Work out the finished part from the listing and answer in its coordinate system (mm). Face numbers are marked on the shaded views. Give positions to 0.01 mm unless a question says otherwise; leave off trailing zeros. Loops run counter-clockwise (first coordinate to the right, second up) from the corner with the lowest first, then second, coordinate; pieces in that order, holes last. Notation, with made-up numbers: (52, -29) - (93, -29) arc R16 cw to (93, -17) - close; hole circle Ø3 at (41.5, 63.5). An arc over 180 degrees is marked (long way). One line per question, with ' | ' between items.
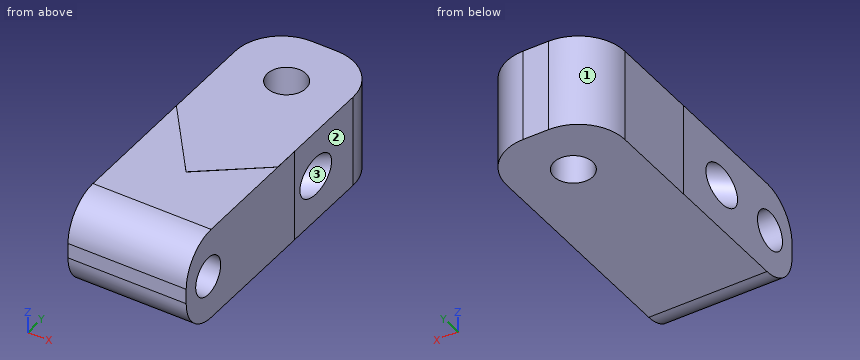
from build123d import *

# Parameters (mm, degrees)
SKETCH5_W           = 60
SKETCH5_H           = 60
SKETCH5_R           = 12.5
BOSS_EXTRUDE3_DEPTH = 25
SKETCH9_R           = 12.5
BOSS_EXTRUDE5_DEPTH = 30
SKETCH10_R          = 12.5
BOSS_EXTRUDE6_DEPTH = 38.21
SKETCH5_2_R         = 12.5
CUT_EXTRUDE2_DEPTH  = 115


with BuildPart() as part:
    # Sketch5 → Boss-Extrude3 (new body, symmetric)
    with BuildSketch(Plane(origin=(0, 0, 0), x_dir=(0, 0, -1), z_dir=(0.789084085, 0.6142852, 0))):
        Rectangle(SKETCH5_W, SKETCH5_H)
        Circle(SKETCH5_R, mode=Mode.SUBTRACT)
    extrude(amount=BOSS_EXTRUDE3_DEPTH, both=True)

    # Sketch9 → Boss-Extrude5 (add, symmetric)
    with BuildSketch(Plane.XY):
        with BuildLine():
            Line((38.155658124, -8.315392543), (38.155658124, 67.179146139))
            ThreePointArc((38.155658124, 67.179146139), (29.368861559, 88.392349575), (8.155658124, 97.179146139))
            Line((8.155658124, 97.179146139), (-8.155658124, 97.179146139))
            ThreePointArc((-8.155658124, 97.179146139), (-29.368861559, 88.392349575), (-38.155658124, 67.179146139))
            Line((-38.155658124, 67.179146139), (-38.155658124, 8.315392543))
            Line((-38.155658124, 8.315392543), (38.155658124, -8.315392543))
        make_face()
        with Locations((0, 59.597275262)):
            Circle(SKETCH9_R, mode=Mode.SUBTRACT)
    extrude(amount=BOSS_EXTRUDE5_DEPTH, both=True)

    # Sketch10 → Boss-Extrude6 (add, symmetric)
    with BuildSketch(Plane(origin=(0, 0, 0), x_dir=(0, 0, -1), z_dir=(1, 0, 0))):
        with BuildLine():
            Line((-4.782552043, -100.050547257), (5, -100.050547257))
            ThreePointArc((5, -100.050547257), (22.67766953, -92.728216787), (30, -75.050547257))
            Line((30, -75.050547257), (30, 8.315392543))
            Line((30, 8.315392543), (-30, 8.315392543))
            Line((-30, 8.315392543), (-29.782467066, -75.115730425))
            ThreePointArc((-29.782467066, -75.115730425), (-22.437160802, -92.751247514), (-4.782552043, -100.050547257))
        make_face()
        with Locations((0.225286959, -78.050547257)):
            Circle(SKETCH10_R, mode=Mode.SUBTRACT)
    extrude(amount=BOSS_EXTRUDE6_DEPTH, both=True)

    # Sketch5_2 → Cut-Extrude2 (cut, symmetric)
    with BuildSketch(Plane(origin=(0, 0, 0), x_dir=(0, 0, -1), z_dir=(0.789084085, 0.6142852, 0))):
        Circle(SKETCH5_2_R)
    extrude(amount=CUT_EXTRUDE2_DEPTH, both=True, mode=Mode.SUBTRACT)


solid = part.part
1. Find section C-C on x = 16. State how many separate pieces and enclosed holes the cut face has, then the cut area to 3 significant figures.
Evaluation:
separate pieces: 1 | enclosed holes: 2 | area: 10,400 mm2
2. Flat-ended cylindrical pins translate along their axes: pin 1 (6 mm diameter, centred on x = -8.5, y = 60, fed in from -Z); pin 2 (3 mm diameter, centred on x = -22, z = 20, fed in from -Y); pin 3 (4 mm diameter, centred on y = 72, z = 13.5, fed in from +X); pin 4 (17.5 mm diameter, centred on y = 45, z = 8.5, fed in from +X). Find the tip coordinate at first contact, or state that the pin passes through.
Evaluation:
pin 1: through | pin 2: y = -95.95 | pin 3: x = 38.02 | pin 4: x = 38.16
3. Determine the mould class of the marked faces 1, 2 and 3 for opening direction X: +X half, -X half, draft (parallel to the pull), parting line (faces both ways), or undercut.
Evaluation:
face 1: -X half | face 2: +X half | face 3: undercut
4. Find section B-B on y = 63. Write down the section's boundary in (x, z), then the cut area to 3 significant figures.
Evaluation:
outline: (-38.16, -30) - (-12.03, -30) - (-12.03, 30) - (-38.16, 30) - close; (12.03, -30) - (38.16, -30) - (38.16, 30) - (12.03, 30) - close | area: 3,140 mm2
5. Find section D-D on z = 17.5. Write down the section's boundary in (x, y).
Evaluation:
outline: (-38.21, -96.57) - (38.21, -96.57) - (38.21, 8.32) - (38.16, 8.32) - (38.16, 67.18) arc R30 ccw to (8.16, 97.18) - (-8.16, 97.18) arc R30 ccw to (-38.16, 67.18) - (-38.16, 8.32) - (-38.21, 8.32) - close; hole circle Ø25 at (0, 59.6)
6. Consider L1, parallel to Y at x = 5, z = 0; L2, parallel to Y at x = 0, z = -5.5; L3, parallel to Y at x = 14, z = -9. Determine where each line is inside the solid, lowest interval first.
Evaluation:
L1: -100.05 to -90.55, -65.55 to -11.95, 19.73 to 48.14, 71.05 to 97.18 | L2: -100.05 to -89.38, -66.72 to -14.23, 14.23 to 47.1, 72.1 to 97.18 | L3: -99.73 to -86.95, -69.15 to -0.09, 21.89 to 96.6
7. Find section A-A on z = -26. Write down the section's boundary in (x, y).
Evaluation:
outline: (-38.21, -88.62) - (38.21, -88.62) - (38.21, 8.32) - (38.16, 8.32) - (38.16, 67.18) arc R30 ccw to (8.16, 97.18) - (-8.16, 97.18) arc R30 ccw to (-38.16, 67.18) - (-38.16, 8.32) - (-38.21, 8.32) - close; hole circle Ø25 at (0, 59.6)
